Could you check a few things on this model? Use its own coordinates, in mm. Give positions to 0.01 mm unless a question says otherwise; leave off trailing zeros. Order: outer loops, then holes, each group sorted by start corner. A loop starts at its lowest first (then second) coordinate and runs counter-clockwise, first axis right, second up. Notation, with made-up numbers: (39, 53.5) - (88, 53.5) arc R18 ccw to (88, 88.5) - close; hole circle Ø1 at (42, 72). An arc over 180 degrees is marked (long way). One line per question, with ' | ' between items. Start each with the question number.
1. Imagine slicing it at C-C (x = -6). Please give me the cut outline in (y, z).
2. Imagine slicing it at D-D (z = 4). Give the number of separate pieces and of enclosed holes in the cut face, and give its area (3 significant figures).
3. Imagine slicing it at B-B (y = 0). Please give me the cut outline in (x, z), and give its area (3 significant figures).
4. Imagine slicing it at A-A (x = 0). Please give me the cut outline in (y, z).
5. I need wall thicknesses on probe 1 along Y at (x, z) = (0, 4.5); probe 2 along X at (y, z) = (15, 2.75); probe 3 along Y at (x, z) = (-8, 2). Which ranges of each line are inside material? Lowest first, please. Write a range as from..to.
6. If we mould it in two halves opening along X, with no side actions, what happens to faces 1 (the cylindrical face through (-2.38, -10.74, 3.45)), 2 (the flat face through (-2, -11, 7)), 3 (the cylindrical face through (-29.97, 1.32, 3.45))? For each: released by +X, released by -X, zero draft, split by the parting line, or undercut.
7. For P1, Ø1.5, axis at x = 18, z = 1.5, coming from the -Y side; P2, Ø4, axis at y = -10, z = 1, coming from the -X side; P3, Ø2, axis at x = 10.5, z = 1.5, coming from the +Y side, each with a flat end and sliding along its axis, tell me the tip position at first contact or that it passes through.
```python
from build123d import *

# Parameters (mm, degrees)
F0_R     = 30
F0_R_2   = 7.5
F0_R_3   = 11
F1_DEPTH = 7


with BuildPart() as f1:
    # F0 (on Top) → F1 (new body)
    with BuildSketch(Plane.XY):
        Circle(F0_R)
        with Locations((-8.677675, -18.019377)):
            Circle(F0_R_2, mode=Mode.SUBTRACT)
        with Locations((-19.498558, -4.450419)):
            Circle(F0_R_2, mode=Mode.SUBTRACT)
        with Locations((8.677675, -18.019377)):
            Circle(F0_R_2, mode=Mode.SUBTRACT)
        with Locations((19.498558, -4.450419)):
            Circle(F0_R_2, mode=Mode.SUBTRACT)
        with Locations((-15.63663, 12.469796)):
            Circle(F0_R_2, mode=Mode.SUBTRACT)
        Circle(F0_R_3, mode=Mode.SUBTRACT)
        with Locations((15.63663, 12.469796)):
            Circle(F0_R_2, mode=Mode.SUBTRACT)
        with Locations((0, 20)):
            Circle(F0_R_2, mode=Mode.SUBTRACT)
    extrude(amount=F1_DEPTH)


solid = f1.part
```
Results found:
1) outline: (-29.39, 0) - (-25.03, 0) - (-25.03, 7) - (-29.39, 7) - close; (-11.01, 0) - (-9.22, 0) - (-9.22, 7) - (-11.01, 7) - close; (9.22, 0) - (15.5, 0) - (15.5, 7) - (9.22, 7) - close; (24.5, 0) - (29.39, 0) - (29.39, 7) - (24.5, 7) - close
2) separate pieces: 1 | enclosed holes: 8 | area: 1,210 mm2
3) outline: (-30, 0) - (-25.54, 0) - (-25.54, 7) - (-30, 7) - close; (-13.46, 0) - (-11, 0) - (-11, 7) - (-13.46, 7) - close; (11, 0) - (13.46, 0) - (13.46, 7) - (11, 7) - close; (25.54, 0) - (30, 0) - (30, 7) - (25.54, 7) - close | area: 97.0 mm2
4) outline: (-30, 0) - (-11, 0) - (-11, 7) - (-30, 7) - close; (11, 0) - (12.5, 0) - (12.5, 7) - (11, 7) - close; (27.5, 0) - (30, 0) - (30, 7) - (27.5, 7) - close
5) probe 1: y = -30..-11, 11..12.5, 27.5..30 | probe 2: x = -25.98..-22.7, -8.58..-5.59, 5.59..8.58, 22.7..25.98 | probe 3: y = -28.91..-25.49, -10.55..-7.55, 7.55..28.91
6) face 1: undercut | face 2: zero draft | face 3: split by the parting line
7) P1: stops at y = -24.54 | P2: stops at x = -28.91 | P3: stops at y = 28.46
